Source: CAD feature listing. Evaluate the final solid. Frame: model axes, mm. A direction names the side the tool comes from. Round coordinates to 2 decimals unless told otherwise and drop trailing zeros. Write each loop counter-clockwise with the first axis right and the second up, starting at its lowest first coordinate (ties: lowest second). Pieces come first, ordered by that corner, then holes. Notation, with made-up numbers: (-23, 5.5) -> (-14, 5.5) arc R11 cw to (-14, 12.5) -> close; hole circle Ø5 at (15.5, -26). An arc over 180 degrees is marked (long way). Put each result on its own line as item: value.
```python
from build123d import *

# Parameters (mm, degrees)
CROQUIS1_W              = 40
CROQUIS1_H              = 20
SALIENTE_EXTRUIR1_DEPTH = 2
CROQUIS3_R              = 0.8
SALIENTE_EXTRUIR2_DEPTH = 4
CROQUIS4_R              = 2.5
CROQUIS4_R_2            = 1
CORTAR_EXTRUIR1_DEPTH   = 0.2
CROQUIS6_R              = 0.8
SALIENTE_EXTRUIR3_DEPTH = 4
CROQUIS10_R             = 2.4
CORTAR_EXTRUIR4_DEPTH   = 2
CORTAR_EXTRUIR5_DEPTH   = 0.3


with BuildPart() as part:
    # Croquis1 → Saliente-Extruir1 (new body)
    with BuildSketch(Plane(origin=(0, 0, 0), x_dir=(1, 0, 0), z_dir=(0, 1, 0))):
        Rectangle(CROQUIS1_W, CROQUIS1_H)
    extrude(amount=SALIENTE_EXTRUIR1_DEPTH)

    # Croquis3 → Saliente-Extruir2 (add)
    with BuildSketch(Plane(origin=(20, 0, 0), x_dir=(0, 0, -1), z_dir=(1, 0, 0))):
        with BuildLine():
            Line((-2.346611166, 8.275044598), (-0.978490727, 21.414260229))
            ThreePointArc((-0.978490727, 21.414260229), (2.899239812, 24.998730722), (6.952577869, 21.614107636))
            Line((6.952577869, 21.614107636), (10, 2))
            Line((10, 2), (-9.308969938, 2))
            ThreePointArc((-9.308969938, 2), (-4.622536743, 3.8002554), (-2.346611166, 8.275044598))
        make_face()
        with Locations((3, 21)):
            Circle(CROQUIS3_R, mode=Mode.SUBTRACT)
    extrude(amount=-SALIENTE_EXTRUIR2_DEPTH)

    # Croquis4 → Cortar-Extruir1 (cut)
    with BuildSketch(Plane.XZ):
        with Locations((7, -5)):
            Circle(CROQUIS4_R)
        with Locations((7, -5)):
            Circle(CROQUIS4_R_2, mode=Mode.SUBTRACT)
        with BuildLine():
            Line((0.5, 8), (0.5, 6))
            ThreePointArc((0.5, 6), (0, 5.5), (-0.5, 6))
            Line((-0.5, 6), (-0.5, 8))
            ThreePointArc((-0.5, 8), (0, 8.5), (0.5, 8))
        make_face()
        with BuildLine():
            Line((2, 8), (2, 6))
            ThreePointArc((2, 6), (2.5, 5.5), (3, 6))
            Line((3, 6), (3, 8))
            ThreePointArc((3, 8), (2.5, 8.5), (2, 8))
        make_face()
        with BuildLine():
            Line((4.5, 8), (4.5, 6))
            ThreePointArc((4.5, 6), (5, 5.5), (5.5, 6))
            Line((5.5, 6), (5.5, 8))
            ThreePointArc((5.5, 8), (5, 8.5), (4.5, 8))
        make_face()
        with BuildLine():
            Line((7, 8), (7, 6))
            ThreePointArc((7, 6), (7.5, 5.5), (8, 6))
            Line((8, 6), (8, 8))
            ThreePointArc((8, 8), (7.5, 8.5), (7, 8))
        make_face()
        with BuildLine():
            Line((9.5, 8), (9.5, 6))
            ThreePointArc((9.5, 6), (10, 5.5), (10.5, 6))
            Line((10.5, 6), (10.5, 8))
            ThreePointArc((10.5, 8), (10, 8.5), (9.5, 8))
        make_face()
        with BuildLine():
            Line((12, 8), (12, 6))
            ThreePointArc((12, 6), (12.5, 5.5), (13, 6))
            Line((13, 6), (13, 8))
            ThreePointArc((13, 8), (12.5, 8.5), (12, 8))
        make_face()
    cortar_extruir1 = extrude(amount=-CORTAR_EXTRUIR1_DEPTH, mode=Mode.SUBTRACT)

    # Simetría2: Cortar-Extruir1 across plane
    add(cortar_extruir1.mirror(Plane(origin=(0, 0, 0), x_dir=(0, 0, 1), z_dir=(1, 0, 0))), mode=Mode.SUBTRACT)

    # Croquis6 → Saliente-Extruir3 (add)
    with BuildSketch(Plane.ZY.offset(20)):
        with BuildLine():
            Line((-10, 2), (-5.943364405, 22.580177542))
            ThreePointArc((-5.943364405, 22.580177542), (-2.929004345, 24.999159819), (-0.032480048, 22.440255986))
            Line((-0.032480048, 22.440255986), (2.113895498, 7.972736033))
            ThreePointArc((2.113895498, 7.972736033), (4.465956479, 3.699488338), (9.03810872, 2))
            Line((9.03810872, 2), (-10, 2))
        make_face()
        with Locations((-3, 22)):
            Circle(CROQUIS6_R, mode=Mode.SUBTRACT)
    extrude(amount=-SALIENTE_EXTRUIR3_DEPTH)

    # Croquis10 → Cortar-Extruir4 (cut)
    with BuildSketch(Plane.ZY.offset(-16)):
        with Locations((-3, 21)):
            Circle(CROQUIS10_R)
    extrude(amount=-CORTAR_EXTRUIR4_DEPTH, mode=Mode.SUBTRACT)

    # Croquis11 → Cortar-Extruir5 (cut)
    with BuildSketch(Plane(origin=(0, 0.47856177, 3.225717872), x_dir=(1, 0, 0), z_dir=(0, 0.146751995, 0.989173317))):
        Polygon((-16.3, 9.076199369), (-17, 9.076199369), (-17, 13.376199369), (-18, 13.376199369), (-18, 14.076199369), (-16.3, 14.076199369), align=None)
        Polygon((-19.7, 9.076199369), (-19.7, 14.076199369), (-19, 14.076199369), (-19, 9.776199369), (-18, 9.776199369), (-18, 9.076199369), align=None)
    extrude(amount=-CORTAR_EXTRUIR5_DEPTH, mode=Mode.SUBTRACT)


solid = part.part
```
Q1. Draft query along X for faces 5 (the flat face through (-7, 0, -5)), 6 (the flat face through (2.5, 0.2, 7)). Return one class per face: +X half, -X half, draft (parallel to the pull), parting line (faces both ways), or undercut.
Ans:
face 5: draft
face 6: undercut
Q2. Pin query (flat end, axial travel): pin 1 (10 mm diameter, centred on x = 7, y = 20.5, fed in from -Z); pin 2 (8 mm diameter, centred on x = 4.5, z = -4, fed in from +Y); pin 3 (0.5 mm diameter, centred on x = -10, z = 7.5, fed in from -Y). Return the tip coordinate at first contact, or that it passes through.
Ans:
pin 1: passes through
pin 2: stops at y = 2
pin 3: stops at y = 0.2
Q3. Reachability of faces 1 (the flat face through (18, 22, -4)), 2 (the cylindrical face through (19.01, 20.29, -3.37)), 3 (the flat face through (-5, 0.2, 7)), 4 (the flat face through (7, 0, -5)) from +Z, -Z, +X, -X, +Y, -Y: full face, straight path, thin tool, end or side. Return the list, or none.
Ans:
face 1: none
face 2: +X
face 3: -Y
face 4: +Z, -Z, +X, -X, -Y
Q4. Cut plane B-B on x = -8.5. Output: boundary loops of the cut face in (y, z).
Ans:
outline: (0, -10) -> (2, -10) -> (2, 10) -> (0, 10) -> (0, -3) -> (0.2, -3) -> (0.2, -7) -> (0, -7) -> close
Q5. Cut plane C-C on y = 4. Output: boundary loops of the cut face in (x, z).
Ans:
outline: (-20, -9.61) -> (-16, -9.61) -> (-16, 4.14) -> (-20, 4.14) -> close; (16, -9.69) -> (20, -9.69) -> (20, 4.41) -> (16, 4.41) -> close
Q6. Cut plane A-A on z = -3. Output: boundary loops of the cut face in (x, y), and give its area (3 significant figures).
Ans:
outline: (-20, 0) -> (-8.5, 0) -> (-8.5, 0.2) -> (-5.5, 0.2) -> (-5.5, 0) -> (5.5, 0) -> (5.5, 0.2) -> (8.5, 0.2) -> (8.5, 0) -> (20, 0) -> (20, 20.2) -> (18, 20.2) -> (18, 18.6) -> (16, 18.6) -> (16, 2) -> (-16, 2) -> (-16, 21.2) -> (-20, 21.2) -> close; (-20, 22.8) -> (-16, 22.8) -> (-16, 25) -> (-20, 25) -> close; (16, 23.4) -> (18, 23.4) -> (18, 21.8) -> (20, 21.8) -> (20, 25) -> (16, 25) -> close
area: 244 mm^2
Q7. Cut plane D-D on x = 12.5. Output: boundary loops of the cut face in (y, z), and give its area (3 significant figures).
Ans:
outline: (0, -10) -> (2, -10) -> (2, 10) -> (0, 10) -> (0, 8.5) -> (0.2, 8.5) -> (0.2, 5.5) -> (0, 5.5) -> close
area: 39.4 mm^2
Q8. Material intervals for line 1 (Y direction, x = 17.55, z = -3); line 2 (X direction, y = 17.5, z = -4); line 3 (Y direction, x = -18.2, z = -3), sorted ascending. Write a range as [from, to].
Ans:
line 1: y = [0, 18.6], [23.4, 25]
line 2: x = [-20, -16], [16, 20]
line 3: y = [0, 21.2], [22.8, 25]
